```python
from build123d import *

# Parameters (mm, degrees)
EXTRUDE1_DEPTH = 90
SKETCH2_R      = 10
EXTRUDE2_DEPTH = 10


with BuildPart() as part:
    # Sketch1 → Extrude1 (new body)
    with BuildSketch(Plane(origin=(0, 0, 0), x_dir=(1, 0, 0), z_dir=(0, 1, 0))):
        with BuildLine():
            Line((0, 40), (0, 30))
            Line((0, 30), (15, 30))
            Line((15, 30), (15, 40))
            Line((15, 40), (30, 40))
            Line((30, 40), (30, 30))
            Line((30, 30), (45, 30))
            Line((45, 30), (45, 40))
            ThreePointArc((45, 40), (85, 0), (45, -40))
            Line((45, -40), (45, -30))
            Line((45, -30), (30, -30))
            Line((30, -30), (30, -40))
            Line((30, -40), (15, -40))
            Line((15, -40), (15, -30))
            Line((15, -30), (0, -30))
            Line((0, -30), (0, -40))
            ThreePointArc((0, -40), (-40, 0), (0, 40))
        make_face()
    extrude(amount=EXTRUDE1_DEPTH)

    # Sketch2 → Extrude2 (add)
    with BuildSketch(Plane(origin=(0, 90, 0), x_dir=(-1, 0, 0), z_dir=(0, 1, 0))):
        with Locations(Location((0, 0, 0), (0, 0, 90))):  # turned: the seam where the file's is
            Circle(SKETCH2_R)
    extrude(amount=EXTRUDE2_DEPTH)


solid = part.part
```
Here's how the part is built. I have some questions about the finished solid (model axes, mm). A direction names the side the tool comes from. Give positions to 0.01 mm unless a question says otherwise; leave off trailing zeros. Order: outer loops, then holes, each group sorted by start corner. A loop starts at its lowest first (then second) coordinate and runs counter-clockwise, first axis right, second up. Notation, with made-up numbers: (49.5, 16.5) - (98.5, 16.5) arc R16 ccw to (98.5, 30.5) - close; hole circle Ø7 at (49.5, -39.5). An arc over 180 degrees is marked (long way). Answer as a JSON object with one key per item and string values. Group by question number.
Item 1: For P1, Ø11, axis at y = 62, z = 33, coming from the -X side; P2, Ø8, axis at y = 26.5, z = 35, coming from the +X side; P3, Ø11, axis at y = 45, z = -33.5, coming from the +X side, each with a flat end and sliding along its axis, tell me the tip position at first contact or that it passes through.
Item 2: If we section it at B-B on z = 0: Please give me the cut outline in (x, y).
Item 3: If we section it at D-D on z = -16: Please give me the cut outline in (x, y), and give its area (3 significant figures).
Item 4: If we section it at A-A on y = 16: Please give me the cut outline in (x, z), and give its area (3 significant figures).
Item 5: If we mould it in two halves opening along X, with no side actions, what happens to faces 4 (the flat face through (37, 44, -30)), 5 (the flat face through (0, 100, 0)), 6 (the cylindrical face through (84.99, 44.37, -0.88))? For each: pulls with the +X half, pulls with the -X half, needs draft (parallel to the pull), parting line crosses it, or undercut.
Item 6: If we section it at C-C on x = 42: Please give me the cut outline in (y, z), and give its area (3 significant figures).
Item 7: Please list where these lines run through material, in increasing order: probe 1 along X at (y, z) = (45.5, 31); probe 2 along X at (y, z) = (8, -36.5); probe 3 along X at (y, z) = (21, -1.5).
Item 8: Which directions (+Z, -Z, +X, -X, +Y, -Y) give clear straight access to the entire face, cutting with the end or side of a thin tool? Please do faces 1 (the flat face through (30, 44, 35)), 2 (the flat face through (15, 44, -35)), 3 (the cylindrical face through (-9.76, 94.93, -2.17)).
Result set:
{
 "1": {"P1": "x = -29.05", "P2": "x = 70.28", "P3": "x = 73.57"},
 "2": {"outline": "(-40, 0) - (85, 0) - (85, 90) - (10, 90) - (10, 100) - (-10, 100) - (-10, 90) - (-40, 90) - close"},
 "3": {"outline": "(-36.66, 0) - (81.66, 0) - (81.66, 90) - (-36.66, 90) - close", "area": "10,600 mm²"},
 "4": {"outline": "(0, -40) - (0, -30) - (15, -30) - (15, -40) - (30, -40) - (30, -30) - (45, -30) - (45, -40) arc R40 ccw to (45, 40) - (45, 30) - (30, 30) - (30, 40) - (15, 40) - (15, 30) - (0, 30) - (0, 40) arc R40 ccw to start", "area": "8,030 mm²"},
 "5": {"face 4": "undercut", "face 5": "needs draft", "face 6": "pulls with the +X half"},
 "6": {"outline": "(0, -30) - (90, -30) - (90, 30) - (0, 30) - close", "area": "5,400 mm²"},
 "7": {"probe 1": "-25.28 to 0, 15 to 30, 45 to 70.28", "probe 2": "-16.36 to 0, 15 to 30, 45 to 61.36", "probe 3": "-39.97 to 84.97"},
 "8": {"face 1": "+Z, +Y, -Y", "face 2": "-Z, +Y, -Y", "face 3": "+Y"}
}
